Build history of the part. All positions in model axes, mm. Face numbers are marked on the shaded views. A direction names the side the tool comes from. Give positions to 0.01 mm unless a question says otherwise; leave off trailing zeros. Order: outer loops, then holes, each group sorted by start corner. A loop starts at its lowest first (then second) coordinate and runs counter-clockwise, first axis right, second up. Notation, with made-up numbers: M -16,79.5 L 2,79.5 A31 ccw 2,112.5 Z; hole C 36.5,-19 d6. An arc over 180 degrees is marked long. One line per item, written item: value.
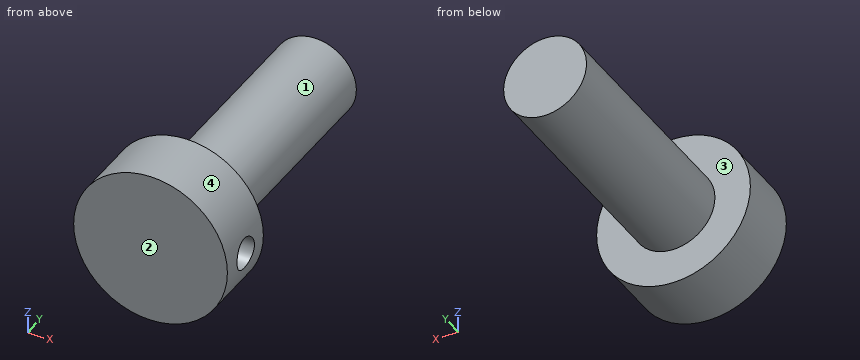
from build123d import *

# Parameters (mm, degrees)
SKETCH2_R           = 11.6
BOSS_EXTRUDE1_DEPTH = 9.8
SKETCH7_R           = 6.25
BOSS_EXTRUDE3_DEPTH = 35
SKETCH3_R           = 2.375
CUT_EXTRUDE1_DEPTH  = 5
SCALE1_SCALE        = 0.8


with BuildPart() as part:
    # Sketch2 → Boss-Extrude1 (new body)
    with BuildSketch(Plane(origin=(0, 0, 0), x_dir=(1, 0, 0), z_dir=(0, 1, 0))):
        with Locations(Location((0, 0, 0), (0, 0, 270))):
            Circle(SKETCH2_R)
    extrude(amount=BOSS_EXTRUDE1_DEPTH)

    # Sketch7 → Boss-Extrude3 (add)
    with BuildSketch(Plane(origin=(0, 9.8, 0), x_dir=(1, 0, 0), z_dir=(0, 1, 0))):
        with Locations(Location((0, 0, 0), (0, 0, 270))):
            Circle(SKETCH7_R)
    extrude(amount=BOSS_EXTRUDE3_DEPTH)

    # Sketch3 → Cut-Extrude1 (cut)
    with BuildSketch(Plane(origin=(11.6, 0, 0), x_dir=(0, 0, -1), z_dir=(1, 0, 0))):
        with Locations((0, 5)):
            Circle(SKETCH3_R)
    extrude(amount=-CUT_EXTRUDE1_DEPTH, mode=Mode.SUBTRACT)


with BuildPart() as part_1:
    # Scale1: scaled about (-0.095056518, 16.420693109, 4.829e-06)
    add(part.part.scale(SCALE1_SCALE).moved(Location((-0.019011304, 3.284138622, 9.66e-07))))


solid = part_1.part
1) Saw through at A-A, the plane z = 0. Write the cut outline in (x, y), then the cut area to 3 significant figures.
Check values:
outline: M -9.3,3.28 L 9.26,3.28 L 9.26,5.38 L 5.26,5.38 L 5.26,9.18 L 9.26,9.18 L 9.26,11.12 L 4.98,11.12 L 4.98,39.12 L -5.02,39.12 L -5.02,11.12 L -9.3,11.12 Z
area: 410 mm^2
2) Tool access for the marked faces 1 and 2: list every direction of +Z, -Z, +X, -X, +Y, -Y with a clear straight run to the whole face (end or side of a thin tool).
Check values:
face 1: +Y
face 2: +Z, -Z, +X, -X, -Y
3) Drill centre lines: probe 1 along Y at (x, z) = (6.35, 0); probe 2 along X at (y, z) = (25.5, 0); probe 3 along Y at (x, z) = (0.25, 8.25). Where is each one in solid material? Low to high. Write a range as from..to.
Check values:
probe 1: 3.28..5.38, 9.18..11.12
probe 2: -5.02..4.98
probe 3: 3.28..11.12
4) Saw through at D-D, the plane y = 8. Write the cut outline in (x, z).
Check values:
outline: M 5.26,-1.76 L 5.26,1.76 L 9.09,1.76 A9.28 ccw long 9.09,-1.76 Z
5) Mould opens along Z. For the marked faces 3 and 4 say: released by +Z, released by -Z, zero draft, split by the parting line, or undercut.
Check values:
face 3: zero draft
face 4: split by the parting line
6) Saw through at C-C, the plane x = -0.75. Write the cut outline in (y, z), then the cut area to 3 significant figures.
Check values:
outline: M 3.28,-9.25 L 11.12,-9.25 L 11.12,-4.95 L 39.12,-4.95 L 39.12,4.95 L 11.12,4.95 L 11.12,9.25 L 3.28,9.25 Z
area: 422 mm^2
7) Saw through at B-B, the plane x = 7.25. Write the cut outline in (y, z).
Check values:
outline: M 3.28,-5.77 L 11.12,-5.77 L 11.12,5.77 L 3.28,5.77 Z; hole C 7.28,0 d3.8
8) Pin check, flat tips, straight feed: pin 1 (5 mm diameter, centred on x = 5, y = 31, fed in from -Z); pin 2 (8 mm diameter, centred on x = -2.5, y = 31, fed in from +Z); pin 3 (4 mm diameter, centred on y = 19.5, z = -6.5, fed in from +X); pin 4 (10 mm diameter, centred on y = 10, z = 1.5, fed in from -X). Stop position of each tip, or through.
Check values:
pin 1: z = -4.32
pin 2: z = 5
pin 3: x = 2.16
pin 4: x = -9.3
